Verification items for the finished model (mm, model axes). Face numbers are marked on the shaded views. A direction names the side the tool comes from. Give positions to 0.01 mm unless a question says otherwise; leave off trailing zeros. Loops run counter-clockwise (first coordinate to the right, second up) from the corner with the lowest first, then second, coordinate; pieces in that order, holes last. Notation, with made-up numbers: (-23, -35.5) - (31, -35.5) arc R7 ccw to (31, -25.5) - close; hole circle Ø3 at (51, 48.5). An arc over 180 degrees is marked (long way). One line per item, written item: value. Start each with the question number.
1. Mould release check, pull along X, two halves, no side actions. Record for the marked faces 1, 2 and 3: pulls with the +X half, pulls with the -X half, needs draft (parallel to the pull), parting line crosses it, or undercut.
2. Access from +Z, -Z, +X, -X, +Y, -Y to the whole of each face (thin tool, end or side, straight path). Record for the marked faces 4, 5 and 6.
3. Sectioned sample at B-B (z = 2.5). Record the cut outline in (x, y).
4. Sectioned sample at D-D (x = 15). Record the cut outline in (y, z).
5. Sectioned sample at C-C (y = 7.5). Record the cut outline in (x, z), plus the area to 3 significant figures.
6. Gauge pin test, flat ends, axial feed: pin 1 (5 mm diameter, centred on x = 21, y = 0, fed in from +Z); pin 2 (5.5 mm diameter, centred on x = -10.5, y = -18.19, fed in from -Z); pin 3 (11.5 mm diameter, centred on x = -3.5, y = 1, fed in from -Z); pin 4 (1 mm diameter, centred on y = -18.5, z = 1.5, fed in from -X). Record the tip position at first contact, or that the pin passes through.
7. Sectioned sample at A-A (x = 0). Record the cut outline in (y, z).
8. Scan lines: L1, parallel to X at y = -1, z = 3.25; L2, parallel to Y at x = -10.5, z = 2.9; L3, parallel to Y at x = 0, z = 1.85. Record each from-to range of solid material in increasing order. Write a range as [from, to].
from build123d import *

# Parameters (mm, degrees)
SKETCH2_R                           = 25
BOSS_EXTRUDE1_DEPTH                 = 7
SKETCH3_R                           = 3.05
DOWEL_PIN_CUTOUT_DEPTH              = 3
MAIN_START                          = -0.5
SKETCH4_R                           = 25.5
SKETCH4_R_2                         = 25
MAIN_HOUSING_BEARING_RETAINER_DEPTH = 0.5
SKETCH5_R                           = 1.55
M3_THRU_DEPTH                       = 37.735541373
SKETCH6_R                           = 3
M3_BUTTON_HEAD_CUTOUT_DEPTH         = 1.7
SKETCH8_R                           = 11.55
INPUT_SHAFT_BEARING_CUTOUT_DEPTH    = 37.735541373
INPUT_START                         = -7
SKETCH9_R                           = 11.55
SKETCH9_R_2                         = 11.05
INPUT_SHAFT_BEARING_RETAINER_DEPTH  = 3


with BuildPart() as part:
    # Sketch2 → Boss-Extrude1 (new body)
    with BuildSketch(Plane.XY):
        Circle(SKETCH2_R)
    extrude(amount=BOSS_EXTRUDE1_DEPTH)

    # Sketch3 → Dowel Pin Cutout (cut)
    with BuildSketch(Plane.XY.offset(7)):
        with Locations((-21, 0)):
            Circle(SKETCH3_R)
        with Locations((-10.5, 18.186533479)):
            Circle(SKETCH3_R)
        with Locations((10.5, 18.186533479)):
            Circle(SKETCH3_R)
        with Locations((21, 0)):
            Circle(SKETCH3_R)
        with Locations((10.5, -18.186533479)):
            Circle(SKETCH3_R)
        with Locations((-10.5, -18.186533479)):
            Circle(SKETCH3_R)
    extrude(amount=-DOWEL_PIN_CUTOUT_DEPTH, mode=Mode.SUBTRACT)

    # Sketch4 → Main Housing Bearing Retainer (add)
    with BuildSketch(Plane.XY.offset(7).offset(MAIN_START)):
        Circle(SKETCH4_R)
        Circle(SKETCH4_R_2, mode=Mode.SUBTRACT)
    extrude(amount=MAIN_HOUSING_BEARING_RETAINER_DEPTH)

    # Sketch5 → M3 Thru (cut, through all)
    with BuildSketch(Plane(origin=(0, 0, 0), x_dir=(-1, 0, 0), z_dir=(0, 0, -1))):
        with Locations((-21, 0)):
            Circle(SKETCH5_R)
        with Locations((-10.5, 18.186533479)):
            Circle(SKETCH5_R)
        with Locations((10.5, 18.186533479)):
            Circle(SKETCH5_R)
        with Locations((21, 0)):
            Circle(SKETCH5_R)
        with Locations((10.5, -18.186533479)):
            Circle(SKETCH5_R)
        with Locations((-10.5, -18.186533479)):
            Circle(SKETCH5_R)
    extrude(amount=-M3_THRU_DEPTH, mode=Mode.SUBTRACT)

    # Sketch6 → M3 Button Head Cutout (cut)
    with BuildSketch(Plane(origin=(0, 0, 0), x_dir=(-1, 0, 0), z_dir=(0, 0, -1))):
        with Locations((-21, 0)):
            Circle(SKETCH6_R)
        with Locations((-10.5, 18.186533479)):
            Circle(SKETCH6_R)
        with Locations((10.5, 18.186533479)):
            Circle(SKETCH6_R)
        with Locations((21, 0)):
            Circle(SKETCH6_R)
        with Locations((10.5, -18.186533479)):
            Circle(SKETCH6_R)
        with Locations((-10.5, -18.186533479)):
            Circle(SKETCH6_R)
    extrude(amount=-M3_BUTTON_HEAD_CUTOUT_DEPTH, mode=Mode.SUBTRACT)

    # Sketch8 → Input Shaft Bearing Cutout (cut, through all)
    with BuildSketch(Plane.XY.offset(7)):
        Circle(SKETCH8_R)
    extrude(amount=-INPUT_SHAFT_BEARING_CUTOUT_DEPTH, mode=Mode.SUBTRACT)

    # Sketch9 → Input Shaft Bearing Retainer (add)
    with BuildSketch(Plane(origin=(0, 0, 0), x_dir=(-1, 0, 0), z_dir=(0, 0, -1)).offset(INPUT_START)):
        with Locations(Location((0, 0, 0), (0, 0, 180))):
            Circle(SKETCH9_R)
        with Locations(Location((0, 0, 0), (0, 0, 180))):
            Circle(SKETCH9_R_2, mode=Mode.SUBTRACT)
    extrude(amount=INPUT_SHAFT_BEARING_RETAINER_DEPTH)


solid = part.part
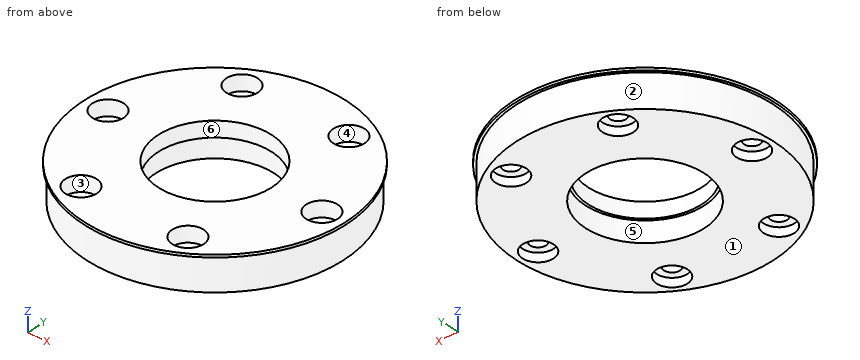
Results are:
1. face 1: needs draft
1. face 2: parting line crosses it
1. face 3: undercut
2. face 4: +Z
2. face 5: -Z
2. face 6: +Z, -Z
3. outline: circle Ø50 at (0, 0); hole circle Ø3.1 at (-21, 0); hole circle Ø3.1 at (-10.5, -18.19); hole circle Ø3.1 at (-10.5, 18.19); hole circle Ø23.1 at (0, 0); hole circle Ø3.1 at (10.5, -18.19); hole circle Ø3.1 at (10.5, 18.19); hole circle Ø3.1 at (21, 0)
4. outline: (-20.62, 6.5) - (-20, 6.5) - (-20, 0) - (20, 0) - (20, 6.5) - (20.62, 6.5) - (20.62, 7) - (-20.62, 7) - close
5. outline: (-24.37, 6.5) - (-23.85, 6.5) - (-23.85, 0) - (-8.78, 0) - (-8.78, 4) - (-8.11, 4) - (-8.11, 7) - (-24.37, 7) - close; (8.11, 4) - (8.78, 4) - (8.78, 0) - (23.85, 0) - (23.85, 6.5) - (24.37, 6.5) - (24.37, 7) - (8.11, 7) - close
5. area: 215 mm^2
6. pin 1: stops at z = 4
6. pin 2: stops at z = 1.7
6. pin 3: passes through
6. pin 4: stops at x = -17.35
7. outline: (-25.5, 6.5) - (-25, 6.5) - (-25, 0) - (-11.55, 0) - (-11.55, 4) - (-11.05, 4) - (-11.05, 7) - (-25.5, 7) - close; (11.05, 4) - (11.55, 4) - (11.55, 0) - (25, 0) - (25, 6.5) - (25.5, 6.5) - (25.5, 7) - (11.05, 7) - close
8. L1: x = [-24.98, -22.18], [-19.82, -11.51], [11.51, 19.82], [22.18, 24.98]
8. L2: y = [-22.69, -19.74], [-16.64, -4.81], [4.81, 16.64], [19.74, 22.69]
8. L3: y = [-25, -11.55], [11.55, 25]
